Geometry check sheet. Reference: the model listing, model coordinates, mm. A direction names the side the tool comes from. Round coordinates to 2 decimals unless told otherwise and drop trailing zeros. Loops run counter-clockwise (first coordinate to the right, second up) from the corner with the lowest first, then second, coordinate; pieces in that order, holes last. Notation, with made-up numbers: M -39,-30 L 15,-30 A29 cw 15,0 Z; hole C 87,19.25 d3. An arc over 180 degrees is marked long. Use one line per item in the form item = value. Start each with the question number.
1. Cross-section at D-D (z = 7.5). Record the boundary of the cut face in (x, y) (3 decimals).
2. Cross-section at B-B (z = 0). Record the boundary of the cut face in (x, y) (3 decimals), then the cut area to 3 significant figures.
3. Draft check along X on faces 3 (the cylindrical face through (9.46, 4.69, 1.05)), 4 (the flat face through (18, 5, 0)), 5 (the flat face through (-0.3, 1.5, 12)). Enter one of: pulls with the +X half, pulls with the -X half, needs draft (parallel to the pull), parting line crosses it, or undercut.
4. Cross-section at A-A (x = 0). Record the boundary of the cut face in (y, z) (3 decimals).
5. Cross-section at C-C (x = 12). Record the boundary of the cut face in (y, z) (3 decimals), then the cut area to 3 significant figures.
6. Set-up check for faces 1 (the flat face through (0, 5, -12)), 2 (the cylindrical face through (-2.54, 3.71, 7)): record each of +Z, -Z, +X, -X, +Y, -Y from which the full face is reachable in a straight line by a thin tool's end or side.
7. Go/stop test with flat-tipped pins: pin 1 (4.5 mm diameter, centred on x = 0, y = 4.765, fed in from +Z); pin 2 (5 mm diameter, centred on x = -12, z = 0, fed in from -Y). Record where each tip stops, or that it passes through.
8. Material ranges on line 1 (Y direction, x = 0, z = 5.5) (3 decimals); line 2 (Z direction, x = 12, y = 6.5); line 3 (X direction, y = 4, z = -2), recorded low to high.
```python
from build123d import *

# Parameters (mm, degrees)
SKETCH1_W                      = 36
SKETCH1_H                      = 24
SKETCH1_R                      = 3.5
BOSS_EXTRUDE1_DEPTH            = 9.53
M5_CLEARANCE_HOLE1_D           = 5.5
M5_CLEARANCE_HOLE1_DEPTH       = 13
M5_CLEARANCE_HOLE1_CSINK_D     = 5.55
M5_CLEARANCE_HOLE1_CSINK_ANGLE = 90
M5_CLEARANCE_HOLE1_TIP         = 1.652366702
M5_CLEARANCE_HOLE2_D           = 5.5
M5_CLEARANCE_HOLE2_DEPTH       = 13
M5_CLEARANCE_HOLE2_CSINK_D     = 5.55
M5_CLEARANCE_HOLE2_CSINK_ANGLE = 90
M5_CLEARANCE_HOLE2_TIP         = 1.652366702


with BuildPart() as part:
    # Sketch1 → Boss-Extrude1 (new body)
    with BuildSketch(Plane(origin=(0, 0, 0), x_dir=(1, 0, 0), z_dir=(0, 1, 0))):
        Rectangle(SKETCH1_W, SKETCH1_H)
        Circle(SKETCH1_R, mode=Mode.SUBTRACT)
    extrude(amount=BOSS_EXTRUDE1_DEPTH)

    # M5 Clearance Hole1
    with Locations(Plane.XY.offset(12)):
        with Locations((0, 4.765)):
            CounterSinkHole(M5_CLEARANCE_HOLE1_D / 2, M5_CLEARANCE_HOLE1_CSINK_D / 2, depth=M5_CLEARANCE_HOLE1_DEPTH, counter_sink_angle=M5_CLEARANCE_HOLE1_CSINK_ANGLE)
            with Locations((0, 0, -(M5_CLEARANCE_HOLE1_DEPTH + M5_CLEARANCE_HOLE1_TIP / 2))):  # 118° drill point
                Cone(0, M5_CLEARANCE_HOLE1_D / 2, M5_CLEARANCE_HOLE1_TIP, mode=Mode.SUBTRACT)

    # M5 Clearance Hole2
    with Locations(Plane(origin=(0, 9.53, 0), x_dir=(1, 0, 0), z_dir=(0, 1, 0))):
        with Locations((12, 0), (-12, 0)):
            CounterSinkHole(M5_CLEARANCE_HOLE2_D / 2, M5_CLEARANCE_HOLE2_CSINK_D / 2, depth=M5_CLEARANCE_HOLE2_DEPTH, counter_sink_angle=M5_CLEARANCE_HOLE2_CSINK_ANGLE)
            with Locations((0, 0, -(M5_CLEARANCE_HOLE2_DEPTH + M5_CLEARANCE_HOLE2_TIP / 2))):  # 118° drill point
                Cone(0, M5_CLEARANCE_HOLE2_D / 2, M5_CLEARANCE_HOLE2_TIP, mode=Mode.SUBTRACT)


solid = part.part
```
Reported:
q1.outline = M -18,0 L 18,0 L 18,9.53 L -18,9.53 Z; hole C 0,4.765 d5.5
q2.outline = M -18,0 L -14.75,0 L -14.75,9.505 L -14.775,9.53 L -18,9.53 Z; M -9.25,0 L -3.5,0 L -3.5,9.53 L -9.225,9.53 L -9.25,9.505 Z; M 3.5,0 L 9.25,0 L 9.25,9.505 L 9.225,9.53 L 3.5,9.53 Z; M 14.75,0 L 18,0 L 18,9.53 L 14.775,9.53 L 14.75,9.505 Z
q2.area = 172 mm²
q3.face_3 = undercut
q3.face_4 = pulls with the +X half
q3.face_5 = needs draft
q4.outline = M 0,-12 L 9.53,-12 L 9.53,-3.5 L 0,-3.5 Z; M 0,3.5 L 2.015,3.5 L 2.015,11.975 L 1.99,12 L 0,12 Z; M 7.515,3.5 L 9.53,3.5 L 9.53,12 L 7.54,12 L 7.515,11.975 Z
q5.outline = M 0,-12 L 9.53,-12 L 9.53,-2.775 L 9.505,-2.75 L 0,-2.75 Z; M 0,2.75 L 9.505,2.75 L 9.53,2.775 L 9.53,12 L 0,12 Z
q5.area = 176 mm²
q6.face_1 = -Z, +X, -X, +Y, -Y
q6.face_2 = +Z
q7.pin_1 = -2.68
q7.pin_2 = through
q8.line_1 = 0 to 2.015, 7.515 to 9.53
q8.line_2 = -12 to -2.75, 2.75 to 12
q8.line_3 = -18 to -13.89, -10.11 to -2.87, 2.87 to 10.11, 13.89 to 18
